Read the model definition and answer for the solid it produces. Units are mm, in the model's axes. Face numbers are marked on the shaded views. A direction names the side the tool comes from. Give positions to 0.01 mm unless a question says otherwise; leave off trailing zeros. Order: outer loops, then holes, each group sorted by start corner. A loop starts at its lowest first (then second) coordinate and runs counter-clockwise, first axis right, second up. Notation, with made-up numbers: (-16, -7.5) - (43, -7.5) arc R15 ccw to (43, -1.5) - close; hole circle Ø10 at (-28.75, 10.25). An arc over 180 degrees is marked (long way). Use a Markdown table: item, result. Add a question column.
1. A cutting plane is placed at C-C on x = -6.25. Determine the outline of the cut face in (y, z) (3 decimals).
2. Flat-ended cylindrical pins translate along their axes: P1, Ø1.1, axis at y = -17.5, z = -9.5, coming from the -X side; P2, Ø0.8, axis at x = -5.5, y = 1.5, coming from the +Z side; P3, Ø4, axis at y = -17.14, z = -14.32, coming from the +X side; P4, Ø1.5, axis at x = -6.5, y = -10, coming from the -Z side. Find the tip coordinate at first contact, or state that the pin passes through.
3. Consider L1, parallel to Z at x = -4.75, y = 1.75; L2, parallel to Y at x = -4.25, z = -13.75; L3, parallel to Y at x = -4.5, z = -9. Determine where each line is inside the solid, lowest interval first.
4. A cutting plane is placed at A-A on z = -13.75. Determine the outline of the cut face in (x, y), and give its area (3 significant figures).
5. Which of the six approach directions +Z, -Z, +X, -X, +Y, -Y give full straight-line access (tool end or side, diameter ignored) to the marked faces 1, 2, 3 and 4?
6. A cutting plane is placed at D-D on z = 2. Determine the outline of the cut face in (x, y).
```python
from build123d import *

# Parameters (mm, degrees)
F1_DEPTH    = 19.05
F3_DEPTH    = 2.54
F5_DEPTH    = 4.445
F6_R        = 1.27
F7_DEPTH    = 25.4
F8_T1_DEPTH = 20.32


# Not quite as in the source:
# - a fillet or chamfer that OpenCascade refuses, or shapes differently, is made with other operations: its cross-section is extruded or revolved along the edge and cut away or added


with BuildPart() as f1:
    # F0 (on Front) → F1 (new body)
    with BuildSketch(Plane.XZ):
        with BuildLine():
            Line((-3.4925, 0), (-3.4925, 8.861606443))
            ThreePointArc((-3.4925, 8.861606443), (-9.525, 0), (-3.4925, -8.861606443))
            Line((-3.4925, -8.861606443), (-3.4925, 0))
        make_face()
    extrude(amount=F1_DEPTH)

    # F2 (on face) → F3 (join)
    with BuildSketch(Plane(origin=(0, 0, 0), x_dir=(-1, 0, 0), z_dir=(0, 1, 0))):
        Polygon((3.7465, 2.54), (3.7465, 0), (3.7465, -2.54), (8.8265, -2.54), (8.8265, 2.54), align=None)
    extrude(amount=F3_DEPTH)

    # F4 (on face) → F5 (join)
    with BuildSketch(Plane.YZ.offset(-3.4925)):
        Polygon((-19.05, -2.0384269301), (-19.05, -8.861606443), (-19.05, -19.779715687), (-15.24, -19.779715687), (-15.24, -8.861606443), (-15.24, -2.0384269301), align=None)
    extrude(amount=-F5_DEPTH)

    # F6 (on face) → F7 (cut)
    with BuildSketch(Plane.YZ.offset(-3.4925)):
        with Locations((-17.145, -14.320661065)):
            Circle(F6_R)
    extrude(amount=-F7_DEPTH, mode=Mode.SUBTRACT)

    # F8: fillet of radius 3.175 on 2 edges, made by hand

    # F8_s2 → F8_t1 (cut)
    with BuildSketch(Plane.YZ.offset(-15.875)):
        with BuildLine():
            ThreePointArc((-15.24, -16.604715687), (-16.1699359697, -18.8497797173), (-18.415, -19.779715687))
            Line((-18.415, -19.779715687), (-15.24, -19.779715687))
            Line((-15.24, -19.779715687), (-15.24, -16.604715687))
        make_face()
        with BuildLine():
            ThreePointArc((-19.05, -16.604715687), (-18.1200640303, -18.8497797173), (-15.875, -19.779715687))
            Line((-15.875, -19.779715687), (-19.05, -19.779715687))
            Line((-19.05, -19.779715687), (-19.05, -16.604715687))
        make_face()
    extrude(amount=F8_T1_DEPTH, mode=Mode.SUBTRACT)


solid = f1.part
```
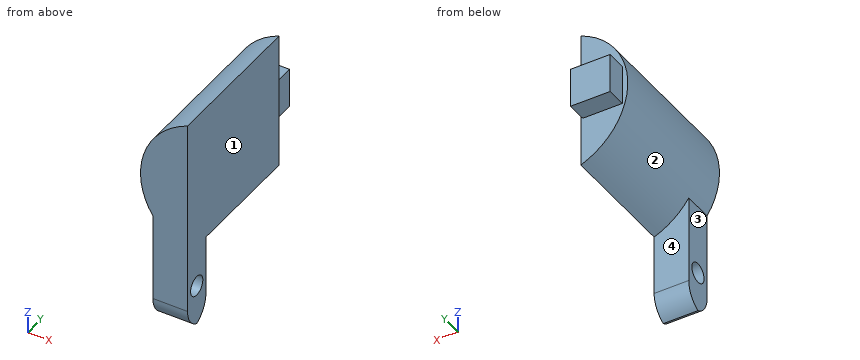
Output values:
| question | item | result |
|---|---|---|
| 1 | outline | (-19.05, -16.605) arc R3.175 ccw to (-17.145, -19.515) arc R3.175 ccw to (-15.24, -16.605) - (-15.24, -7.188) - (0, -7.188) - (0, -2.54) - (2.54, -2.54) - (2.54, 2.54) - (0, 2.54) - (0, 7.188) - (-19.05, 7.188) - close; hole circle Ø2.54 at (-17.145, -14.321) |
| 2 | P1 | x = -7.94 |
| 2 | P2 | z = 2.54 |
| 2 | P3 | x = -3.49 |
| 2 | P4 | z = -7.59 |
| 3 | L1 | -2.54 to 2.54 |
| 3 | L2 | -19.05 to -18.28, -16.01 to -15.24 |
| 3 | L3 | -19.05 to -15.24 |
| 4 | outline | (-7.94, -19.05) - (-3.49, -19.05) - (-3.49, -18.28) - (-7.94, -18.28) - close; (-7.94, -16.01) - (-3.49, -16.01) - (-3.49, -15.24) - (-7.94, -15.24) - close |
| 4 | area | 6.85 mm² |
| 5 | face 1 | +Z, -Z, +X, +Y, -Y |
| 5 | face 2 | -X, +Y |
| 5 | face 3 | -Z, -X, +Y, -Y |
| 5 | face 4 | -Z, -X, +Y |
| 6 | outline | (-9.31, -19.05) - (-3.49, -19.05) - (-3.49, 0) - (-3.75, 0) - (-3.75, 2.54) - (-8.83, 2.54) - (-8.83, 0) - (-9.31, 0) - close |
